CAD build for the part. Positions are in the model's coordinates, mm. A direction names the side the tool comes from. Coordinates: 2 decimals unless noted, no trailing zeros. Write each loop counter-clockwise with the first axis right and the second up, starting at its lowest first coordinate (ties: lowest second). Pieces come first, ordered by that corner, then holes. Notation, with made-up numbers: (14, 11) -> (62, 11) arc R25 ccw to (62, 25) -> close; hole circle Ø6 at (60.25, -31). An arc over 180 degrees is marked (long way). Answer as CSV lines item,"result".
```python
from build123d import *

# Parameters (mm, degrees)
BOSS_EXTRUDE1_DEPTH = 3
SKETCH2_W           = 4
SKETCH2_H           = 15.5
BOSS_EXTRUDE2_DEPTH = 1
CUT_EXTRUDE1_DEPTH  = 0.25
CUT_EXTRUDE7_DEPTH  = 6


with BuildPart() as part:
    # Sketch1 → Boss-Extrude1 (new body)
    with BuildSketch(Plane(origin=(0, 0, 0), x_dir=(1, 0, 0), z_dir=(0, 1, 0))):
        Polygon((-1, -7.25), (1, -7.25), (1, 7.25), (2, 7.25), (2, -7.25), (2, -8.25), (1, -8.25), (-2, -8.25), (-2, 7.25), (-1, 7.25), align=None)
    extrude(amount=BOSS_EXTRUDE1_DEPTH)

    # Sketch2 → Boss-Extrude2 (add)
    with BuildSketch(Plane(origin=(0, 3, 0), x_dir=(1, 0, 0), z_dir=(0, 1, 0))):
        with Locations((0, -0.5)):
            Rectangle(SKETCH2_W, SKETCH2_H)
    extrude(amount=BOSS_EXTRUDE2_DEPTH)

    # Sketch3 → Cut-Extrude1 (cut)
    with BuildSketch(Plane.XZ):
        Polygon((-1, 7.25), (1, 7.25), (1, -7.25), (1.5, -7.25), (1.5, 7.717200742), (-1.5, 7.717200742), (-1.5, -7.25), (-1, -7.25), align=None)
    extrude(amount=-CUT_EXTRUDE1_DEPTH, mode=Mode.SUBTRACT)

    # Sketch9 → Cut-Extrude7 (cut)
    with BuildSketch(Plane(origin=(31.168539268, -3, 26.546214854), x_dir=(-0.7071067811865431, 0, 0.7071067811865519), z_dir=(0, -1, 0))):
        Polygon((7.620004071, 34.212873731), (9.865582661, 36.458452321), (9.847893929, 36.476141053), (-10.673980141, 56.998015123), (-12.919044171, 54.752951093), (7.602829899, 34.231077023), align=None)
    extrude(amount=-CUT_EXTRUDE7_DEPTH, mode=Mode.SUBTRACT)


solid = part.part
```
Item 1: Saw through at A-A on z = -2.5. Give the cut face in (x, y).
Answer below:
outline,"(-2, 0) -> (-1.59, 0) -> (-1.59, 3) -> (1.59, 3) -> (1.59, 0) -> (2, 0) -> (2, 4) -> (-2, 4) -> close"
Item 2: Flat gauge pins, fed straight in: pin 1 (2 mm diameter, centred on x = -1, z = -1, fed in from -Y); pin 2 (0.9 mm diameter, centred on x = -0.5, y = 2, fed in from -Z). Where does each tip first touch, or does it go through?
Answer below:
pin 1,"stops at y = 0"
pin 2,"stops at z = 7.74"
Item 3: Wall check: line 1 (X direction, y = 2.9, z = -2.5); line 2 (Z direction, x = 0.4, y = 0.3); line 3 (Y direction, x = -1.25, z = 4.25). Give the ranges that are in metal, low to high. Write a range as from..to.
Answer below:
line 1,"x = -2..-1.59, 1.59..2"
line 2,"z = 7.74..8.25"
line 3,"y = 3..4"
Item 4: Two-plate mould, pull along X, no slides. Class faces 3 (the flat face through (0, 2, 8.25)), 4 (the flat face through (1.587, 1, 0)), 5 (the flat face through (-2, 2, 1)): pulls with the +X half, pulls with the -X half, needs draft (parallel to the pull), parting line crosses it, or undercut.
Answer below:
face 3,"needs draft"
face 4,"undercut"
face 5,"pulls with the -X half"
Item 5: Saw through at B-B on x = 1.25. Give the cut face in (y, z).
Answer below:
outline,"(0, 7.74) -> (3, 7.74) -> (3, -7.25) -> (4, -7.25) -> (4, 8.25) -> (0, 8.25) -> close"
Item 6: 3-axis set-ups, long thin cutter, end or side, ignore diameter. For faces 1 (the flat face through (0, 3, 1)), 2 (the flat face through (-1.8, 0, 1)): which of +Z, -Z, +X, -X, +Y, -Y reach the whole face in a straight line?
Answer below:
face 1,"-Z, -Y"
face 2,"+Z, -Z, +X, -X, -Y"
